from build123d import *

# Parameters (mm, degrees)
SKETCH_1_W          = 33
SKETCH_1_H          = 16
EXTRUDE_1_DEPTH     = 8.5
SKETCH_4_R          = 1.6
EXTRUDE_2_DEPTH     = 6
FILLET_1_R          = 10
SKETCH_5_W          = 8.5
SKETCH_5_H          = 6
EXTRUDE_3_DEPTH     = 33
CUT_EXTRUDE_1_REACH = 38.991
SKETCH_6_W          = 9.13
SKETCH_6_H          = 3
FILLET_2_R          = 1


with BuildPart() as part:
    # Sketch 1 → Extrude 1 (new body)
    with BuildSketch(Plane.XY):
        Rectangle(SKETCH_1_W, SKETCH_1_H)
    extrude(amount=-EXTRUDE_1_DEPTH)

    # Sketch 3 → Cut-Revolve 1 (revolve, cut)
    with BuildSketch(Plane(origin=(0, 0, 0), x_dir=(1, 0, 0), z_dir=(0, 1, 0)), mode=Mode.PRIVATE) as cut_revolve_1_sk:
        Polygon((-7, 0), (-7, 6.1), (-8.578163358, 6.1), (-12.1, 0), align=None)
    cut_revolve_1 = revolve(cut_revolve_1_sk.sketch.rotate(Axis((-7, 0, 0), (0, 0, -1)), 180), axis=Axis((-7, 0, 0), (0, 0, -1)), mode=Mode.SUBTRACT)

    # Mirror 1: Cut-Revolve 1 across plane
    add(cut_revolve_1.mirror(Plane(origin=(0, 0, 0), x_dir=(0, 0, 1), z_dir=(1, 0, 0))), mode=Mode.SUBTRACT)

    # Fillet 1
    fillet_1_edges = [part.edges().sort_by_distance(p)[0] for p in [
        (16.5, -8, -4.25),
        (-16.5, -8, -4.25),
    ]]
    fillet(fillet_1_edges, radius=FILLET_1_R)



with BuildPart() as body_2:
    # Sketch 4 → Extrude 2 (new body)
    with BuildSketch(Plane(origin=(0, 8, 0), x_dir=(1, 0, 0), z_dir=(0, 1, 0))):
        Polygon((-16.5, 0), (-10.5, 0), (6.5, 0), (16.5, 0), (16.5, -9.13), (-16.5, -9.13), align=None)
        with Locations(Location((-6.25, -6.13, 0), (0, 0, 270))):
            Circle(SKETCH_4_R, mode=Mode.SUBTRACT)
        with Locations(Location((2.25, -6.13, 0), (0, 0, 270))):
            Circle(SKETCH_4_R, mode=Mode.SUBTRACT)
    extrude(amount=EXTRUDE_2_DEPTH)


with BuildPart() as part_1:
    add(part.part)

    add(body_2.part)  # Extrude 3 merges body 2
    # Sketch 5 → Extrude 3 (add)
    with BuildSketch(Plane(origin=(16.5, 0, 0), x_dir=(0, 0, -1), z_dir=(1, 0, 0))):
        with Locations((4.25, 11)):
            Rectangle(SKETCH_5_W, SKETCH_5_H)
    extrude(amount=-EXTRUDE_3_DEPTH)

    # Sketch 6 → Cut-Extrude 1 (cut, up to next)
    with BuildSketch(Plane(origin=(16.5, 0, 0), x_dir=(0, 0, -1), z_dir=(1, 0, 0)), mode=Mode.PRIVATE) as cut_extrude_1_sk1:
        with Locations((-4.565, 9.5)):
            Rectangle(SKETCH_6_W, SKETCH_6_H)
    cut_extrude_1_tool1 = extrude(cut_extrude_1_sk1.sketch, amount=-CUT_EXTRUDE_1_REACH, mode=Mode.PRIVATE) & part_1.part
    add(cut_extrude_1_tool1.solids().sort_by_distance((16.5, 9.5, 4.565))[0], mode=Mode.SUBTRACT)

    # Fillet 2
    fillet_2_edges = [part_1.edges().sort_by_distance(p)[0] for p in [
        (-16.5, 12.5, 9.13),
        (16.5, 12.5, 9.13),
        (0, 11, 0),
    ]]
    fillet(fillet_2_edges, radius=FILLET_2_R)


solid = part_1.part
Geometry: final body of the model. Coordinates: model frame, mm. A direction names the side the tool comes from. Coordinates: 2 decimals unless noted, no trailing zeros. Order: outer loops, then holes, each group sorted by start corner. A loop starts at its lowest first (then second) coordinate and runs counter-clockwise, first axis right, second up.
1) Set-up query: faces 4 (the flat face through (7, 0, -6.1)), 5 (the flat face through (0, 3, 0)), 6 (the flat face through (16.5, 9, -2)). Return all of +Z, -Z, +X, -X, +Y, -Y with unobstructed straight access to the full face (end or side cutting, diameter ignored); none if empty.
Result sheet:
face 4: +Z
face 5: +Z, +X, -X, -Y
face 6: +Z, -Z, +X, +Y, -Y
2) Section C-C (z = -7.5). Return loops of the section in (x, y), then the cut area to 3 significant figures.
Result sheet:
outline: (-16.5, 2) arc R10 ccw to (-6.5, -8) - (6.5, -8) arc R10 ccw to (16.5, 2) - (16.5, 14) - (-16.5, 14) - close
area: 683 mm2
3) Section D-D (z = -0.75). Return loops of the section in (x, y), then the cut area to 3 significant figures.
Result sheet:
outline: (-16.5, 2) arc R10 ccw to (-6.5, -8) - (6.5, -8) arc R10 ccw to (16.5, 2) - (16.5, 14) - (-16.5, 14) - close; hole circle Ø9.33 at (-7, 0); hole circle Ø9.33 at (7, 0)
area: 546 mm2
4) Section B-B (x = 1.5). Return loops of the section in (y, z).
Result sheet:
outline: (-8, -8.5) - (14, -8.5) - (14, 4.72) - (11, 4.72) - (11, 1) arc R1 cw to (10, 0) - (-8, 0) - close; (11, 7.54) - (14, 7.54) - (14, 9.13) - (11, 9.13) - close
5) Section A-A (z = 6.13). Return loops of the section in (x, y), then the cut area to 3 significant figures.
Result sheet:
outline: (-16.5, 11) - (-7.85, 11) - (-7.85, 14) - (-16.5, 14) - close; (-4.65, 11) - (0.65, 11) - (0.65, 14) - (-4.65, 14) - close; (3.85, 11) - (16.5, 11) - (16.5, 14) - (3.85, 14) - close
area: 79.8 mm2
6) Ray query, probe 1 along X at (y, z) = (11.9, 6.13); probe 2 along Z at (x, y) = (-6.25, 12.65); probe 3 along X at (y, z) = (12.5, 7.5). Return the intervals inside material, ascending.
Result sheet:
probe 1: x = -16.5 to -7.85, -4.65 to 0.65, 3.85 to 16.5
probe 2: z = -8.5 to 4.53, 7.73 to 9.13
probe 3: x = -16.5 to -7.08, -5.42 to 1.42, 3.08 to 16.5
7) Draft query along Z for faces 1 (the cylindrical face through (13.49, -5.15, -4.31)), 2 (the cylindrical face through (-0.231, 10.699, 0.285)), 3 (the cylindrical face through (-7.22, 12.48, 4.86)). Return one class per face: released by +Z, released by -Z, zero draft, split by the parting line, or undercut.
Result sheet:
face 1: zero draft
face 2: released by +Z
face 3: undercut
8) First-contact query: P1, Ø9, axis at x = -3.5, z = 3.5, coming from the -Y side; P2, Ø8, axis at y = -4, z = 1, coming from the +X side; P3, Ø6, axis at y = -3.5, z = -5.5, coming from the -X side; P4, Ø2.5, axis at x = 6.5, y = 0.5, coming from the +Z side. Flat tips, straight axial feed; report the tip coordinate or a pass-through.
Result sheet:
P1: stops at y = -8
P2: stops at x = 16.27
P3: stops at x = -16.18
P4: stops at z = -5.44
